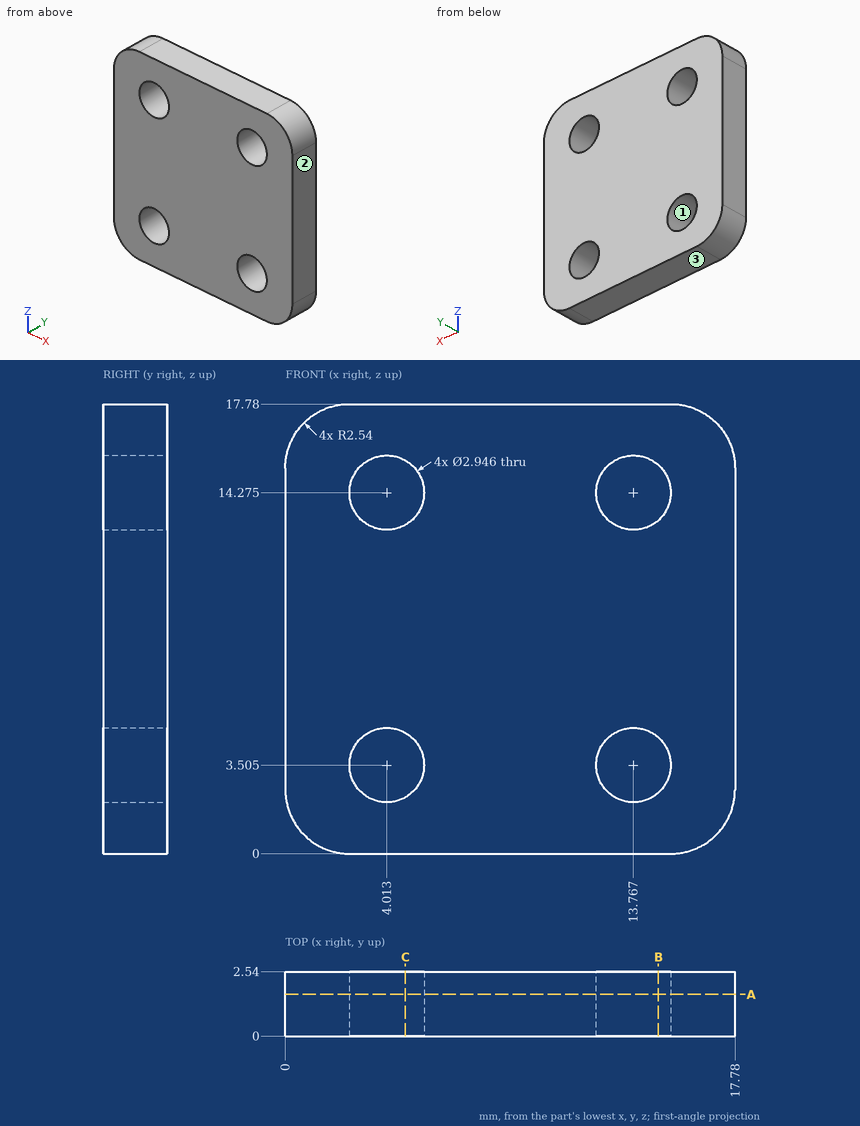
Geometry check sheet. Reference: drawing and pictorial views, mm from the part's lowest x, y, z. Round coordinates to 2 decimals unless told otherwise and drop trailing zeros. Order: outer loops, then holes, each group sorted by start corner. A loop starts at its lowest first (then second) coordinate and runs counter-clockwise, first axis right, second up. Notation, with made-up numbers: M 16,-26.75 L 64,-26.75 A19 cw 64,10.25 Z; hole C 28,25.25 d2. An arc over 180 degrees is marked long. Write item = value, one per line.
Q1. Release check for a two-part mould opening along X. For the marked faces 1, 2 and 3 record: released by +X, released by -X, zero draft, split by the parting line, or undercut.
Answer block:
face_1 = undercut
face_2 = released by +X
face_3 = zero draft
Q2. Depth check by flat-ended pin: pin 1 Ø2 at (x, z) = (9.5, 11.5) entering from -Y. Enter the tip coordinate at first touch or a pass-through.
Answer block:
pin_1 = 0
Q3. Section check A-A (y = 1.65). Enter the section's corners in (x, z) (1 decimal).
Answer block:
outline = M 0,2.5 A2.5 ccw 2.5,0 L 15.2,0 A2.5 ccw 17.8,2.5 L 17.8,15.2 A2.5 ccw 15.2,17.8 L 2.5,17.8 A2.5 ccw 0,15.2 Z; hole C 4,3.5 d2.9; hole C 4,14.3 d2.9; hole C 13.8,3.5 d2.9; hole C 13.8,14.3 d2.9
Q4. Section check B-B (x = 14.75). Enter the section's corners in (y, z).
Answer block:
outline = M 0,0 L 2.54,0 L 2.54,2.41 L 0,2.41 Z; M 0,4.6 L 2.54,4.6 L 2.54,13.18 L 0,13.18 Z; M 0,15.37 L 2.54,15.37 L 2.54,17.78 L 0,17.78 Z
Q5. Section check C-C (x = 4.75). Enter the section's corners in (y, z).
Answer block:
outline = M 0,0 L 2.54,0 L 2.54,2.23 L 0,2.23 Z; M 0,4.78 L 2.54,4.78 L 2.54,13 L 0,13 Z; M 0,15.55 L 2.54,15.55 L 2.54,17.78 L 0,17.78 Z
Q6. Scan lines: line 1 (Z direction, x = 4, y = 1.1); line 2 (Z direction, x = 3, y = 1.75) (1 decimal); line 3 (X direction, y = 0.2, z = 14) (1 decimal). Record each from-to range of solid material in increasing order.
Answer block:
line_1 = 0 to 2.03, 4.98 to 12.8, 15.75 to 17.78
line_2 = 0 to 2.4, 4.6 to 13.2, 15.3 to 17.8
line_3 = 0 to 2.6, 5.5 to 12.3, 15.2 to 17.8
